```python
from build123d import *

# Parameters (mm, degrees)
SKETCH1_W           = 26.3
SKETCH1_H           = 14
SKETCH1_W_2         = 21.3
SKETCH1_H_2         = 9
EXTRUDE_THIN1_DEPTH = 4.5
SKETCH2_W           = 26.3
SKETCH2_H           = 14
BOSS_EXTRUDE1_DEPTH = 5.8
SKETCH3_W           = 26.3
SKETCH3_H           = 14
BOSS_EXTRUDE2_DEPTH = 2
SKETCH4_W           = 4.5
SKETCH4_H           = 21.3
CUT_EXTRUDE1_DEPTH  = 18
CUT_EXTRUDE4_DEPTH  = 4
SKETCH8_W           = 21.3
SKETCH8_H           = 11.5
BOSS_EXTRUDE3_DEPTH = 1.4
SKETCH5_R           = 1.85
CUT_EXTRUDE2_DEPTH  = 10
SKETCH9_W           = 12.3
SKETCH9_H           = 14
BOSS_EXTRUDE4_DEPTH = 1.5
CHAMFER1_SIZE       = 3


with BuildPart() as part:
    # Sketch1 → Extrude-Thin1 (new body)
    with BuildSketch(Plane.YZ):
        with Locations((10.65, 4.5)):
            Rectangle(SKETCH1_W, SKETCH1_H)
        with Locations((10.65, 4.5)):
            Rectangle(SKETCH1_W_2, SKETCH1_H_2, mode=Mode.SUBTRACT)
    extrude(amount=EXTRUDE_THIN1_DEPTH)

    # Sketch2 → Boss-Extrude1 (add)
    with BuildSketch(Plane.YZ.offset(4.5)):
        with Locations((10.65, 4.5)):
            Rectangle(SKETCH2_W, SKETCH2_H)
    extrude(amount=BOSS_EXTRUDE1_DEPTH)

    # Sketch3 → Boss-Extrude2 (add)
    with BuildSketch(Plane(origin=(0, 0, 0), x_dir=(0, -1, 0), z_dir=(-1, 0, 0))):
        with Locations((-10.65, 4.5)):
            Rectangle(SKETCH3_W, SKETCH3_H)
    extrude(amount=BOSS_EXTRUDE2_DEPTH)

    # Sketch4 → Cut-Extrude1 (cut)
    with BuildSketch(Plane(origin=(0, 0, 9), x_dir=(1, 0, 0), z_dir=(0, 0, -1))):
        with Locations((2.25, -10.65)):
            Rectangle(SKETCH4_W, SKETCH4_H)
    extrude(amount=-CUT_EXTRUDE1_DEPTH, mode=Mode.SUBTRACT)

    # Sketch7 → Cut-Extrude4 (cut)
    with BuildSketch(Plane(origin=(4.5, 0, 0), x_dir=(0, -1, 0), z_dir=(-1, 0, 0))):
        Polygon((-14.85, 6.279660954), (-14.85, 11.5), (-9.15, 11.5), (-9.15, 6.691276574), (-9.15, 1.854551733), (-12, 0.209103466), (-14.85, 1.854551733), align=None)
        Polygon((-6.85, 1.854551733), (-4, 0.209103466), (-1.15, 1.854551733), (-1.15, 5.098904977), (-1.15, 11.5), (-6.85, 11.5), (-6.85, 5.026706695), align=None)
    extrude(amount=-CUT_EXTRUDE4_DEPTH, mode=Mode.SUBTRACT)

    # Sketch8 → Boss-Extrude3 (add)
    with BuildSketch(Plane(origin=(4.5, 0, 0), x_dir=(0, -1, 0), z_dir=(-1, 0, 0))):
        with Locations((-10.65, 5.75)):
            Rectangle(SKETCH8_W, SKETCH8_H)
    extrude(amount=-BOSS_EXTRUDE3_DEPTH)

    # Sketch5 → Cut-Extrude2 (cut)
    with BuildSketch(Plane.YZ.offset(10.3)):
        with Locations(Location((4, 3.5, 0), (0, 0, 270))):
            Circle(SKETCH5_R)
        with Locations(Location((12, 3.5, 0), (0, 0, 270))):
            Circle(SKETCH5_R)
    extrude(amount=-CUT_EXTRUDE2_DEPTH, mode=Mode.SUBTRACT)

    # Sketch9 → Boss-Extrude4 (add)
    with BuildSketch(Plane(origin=(0, 23.8, 0), x_dir=(-1, 0, 0), z_dir=(0, 1, 0))):
        with Locations((-4.15, 4.5)):
            Rectangle(SKETCH9_W, SKETCH9_H)
    extrude(amount=BOSS_EXTRUDE4_DEPTH)

    # Chamfer1
    chamfer1_edges = [part.edges().sort_by_distance(p)[0] for p in [
        (10.3, 25.3, 4.5),
        (10.3, -2.5, 4.5),
    ]]
    chamfer(chamfer1_edges, length=CHAMFER1_SIZE)


solid = part.part
```
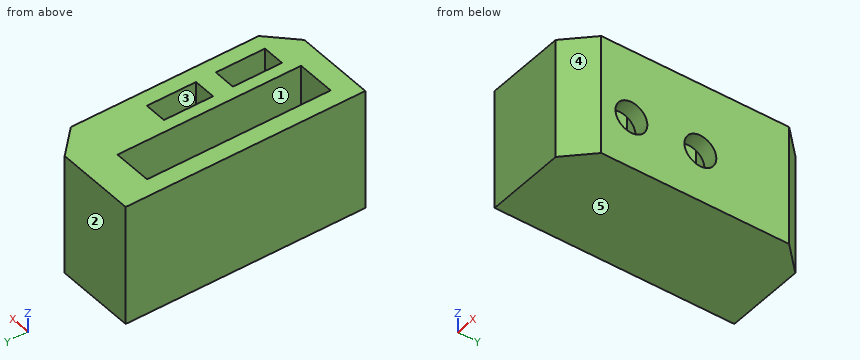
Build history of the part. All positions in model axes, mm. Face numbers are marked on the shaded views. A direction names the side the tool comes from. Round coordinates to 2 decimals unless told otherwise and drop trailing zeros. Write each loop counter-clockwise with the first axis right and the second up, starting at its lowest first coordinate (ties: lowest second). Pieces come first, ordered by that corner, then holes.
1) 3-axis set-ups, long thin cutter, end or side, ignore diameter. For the marked faces 1 and 2: which of +Z, -Z, +X, -X, +Y, -Y reach the whole face in a straight line?
2) Band-saw the part on D-D, the plane z = -0.5. List the corners of the cut face in (x, y), and give its area (3 significant figures).
3) Mould opens along X. For the marked faces 3, 4 and 5 say: +X half, -X half, draft (parallel to the pull), parting line (faces both ways), or undercut.
4) Band-saw the part on B-B, the plane x = 6.5. List the corners of the cut face in (y, z), and give its area (3 significant figures).
5) Pin check, flat tips, straight feed: pin 1 (3.5 mm diameter, centred on y = 4, z = 3.5, fed in from +X); pin 2 (1.3 mm diameter, centred on x = 1.5, y = 10, fed in from +Z). Stop position of each tip, or through.
6) Drill centre lines: probe 1 along Y at (x, z) = (5.35, 3.5); probe 2 along X at (y, z) = (13.5, 2.25); probe 3 along Y at (x, z) = (5.5, 5). Where is each one in solid material? Low to high.
7) Band-saw the part on C-C, the plane y = 17. List the corners of the cut face in (x, z), and give its area (3 significant figures).
Ans:
1. face 1: +Z
1. face 2: +Z, -Z, +X, -X, +Y
2. outline: (-2, -2.5) - (7.3, -2.5) - (10.3, 0.5) - (10.3, 22.3) - (7.3, 25.3) - (-2, 25.3) - close
2. area: 333 mm2
3. face 3: undercut
3. face 4: +X half
3. face 5: draft
4. outline: (-2.5, -2.5) - (25.3, -2.5) - (25.3, 11.5) - (14.85, 11.5) - (14.85, 1.85) - (12, 0.21) - (9.15, 1.85) - (9.15, 11.5) - (6.85, 11.5) - (6.85, 1.85) - (4, 0.21) - (1.15, 1.85) - (1.15, 11.5) - (-2.5, 11.5) - close
4. area: 270 mm2
5. pin 1: stops at x = 0
5. pin 2: stops at z = 0
6. probe 1: y = -2.5 to 2.15, 5.85 to 10.15, 13.85 to 25.3
6. probe 2: x = -2 to 0, 4.5 to 5.9, 8.5 to 10.3
6. probe 3: y = -2.5 to 2.92, 5.08 to 10.92, 13.08 to 25.3
7. outline: (-2, -2.5) - (10.3, -2.5) - (10.3, 11.5) - (4.5, 11.5) - (4.5, 0) - (0, 0) - (0, 11.5) - (-2, 11.5) - close
7. area: 120 mm2
